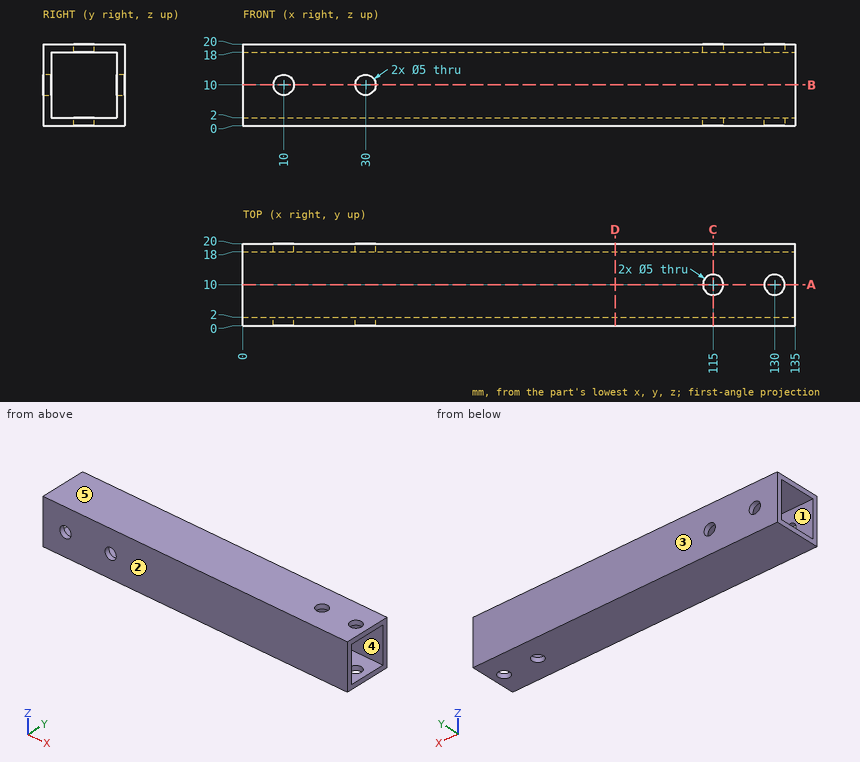
The drawing under review shows one solid part. Ordinate dimensions are in mm from its lowest x, y, z. A direction names the side the tool comes from. Round coordinates to 2 decimals unless told otherwise and drop trailing zeros. Order: outer loops, then holes, each group sorted by start corner. A loop starts at its lowest first (then second) coordinate and runs counter-clockwise, first axis right, second up. Notation, with made-up numbers: (85.5, -35) -> (111.5, -35) arc R20 ccw to (111.5, -23) -> close; hole circle Ø10 at (55.5, 44.25). An arc over 180 degrees is marked (long way). Use a Markdown table: item, result.
Q1. Tool access review of the marked faces 4 and 5: name each direction out of +Z, -Z, +X, -X, +Y, -Y from which nothing blocks a thin tool from reaching the whole face with its end or side.
Values:
| item | result |
|---|---|
| face 4 | +X, -X |
| face 5 | +Z, +X, -X, +Y, -Y |
Q2. Mouldability with a two-part tool opening along Y and no side actions: class the marked faces 1, 2 and 3 as +Y half, -Y half, draft (parallel to the pull), parting line (faces both ways), or undercut.
Values:
| item | result |
|---|---|
| face 1 | undercut |
| face 2 | -Y half |
| face 3 | +Y half |
Q3. We need section A-A on y = 10. Write out the cut boundary in (x, z), then the cut area to 3 significant figures.
Values:
| item | result |
|---|---|
| outline | (0, 0) -> (112.5, 0) -> (112.5, 2) -> (0, 2) -> close; (0, 18) -> (112.5, 18) -> (112.5, 20) -> (0, 20) -> close; (117.5, 0) -> (127.5, 0) -> (127.5, 2) -> (117.5, 2) -> close; (117.5, 18) -> (127.5, 18) -> (127.5, 20) -> (117.5, 20) -> close; (132.5, 0) -> (135, 0) -> (135, 2) -> (132.5, 2) -> close; (132.5, 18) -> (135, 18) -> (135, 20) -> (132.5, 20) -> close |
| area | 500 mm^2 |
Q4. We need section C-C on x = 115. Write out the cut boundary in (y, z), then the cut area to 3 significant figures.
Values:
| item | result |
|---|---|
| outline | (0, 0) -> (7.5, 0) -> (7.5, 2) -> (2, 2) -> (2, 18) -> (7.5, 18) -> (7.5, 20) -> (0, 20) -> close; (12.5, 0) -> (20, 0) -> (20, 20) -> (12.5, 20) -> (12.5, 18) -> (18, 18) -> (18, 2) -> (12.5, 2) -> close |
| area | 124 mm^2 |
Q5. We need section B-B on z = 10. Write out the cut boundary in (x, y), then the cut area to 3 significant figures.
Values:
| item | result |
|---|---|
| outline | (0, 0) -> (7.5, 0) -> (7.5, 2) -> (0, 2) -> close; (0, 18) -> (7.5, 18) -> (7.5, 20) -> (0, 20) -> close; (12.5, 0) -> (27.5, 0) -> (27.5, 2) -> (12.5, 2) -> close; (12.5, 18) -> (27.5, 18) -> (27.5, 20) -> (12.5, 20) -> close; (32.5, 0) -> (135, 0) -> (135, 2) -> (32.5, 2) -> close; (32.5, 18) -> (135, 18) -> (135, 20) -> (32.5, 20) -> close |
| area | 500 mm^2 |
Q6. For line 1 (X direction, y = 19.35, z = 10); line 2 (Y direction, x = 129, z = 7), list the stretches that pass through material, from the lowest coordinate up.
Values:
| item | result |
|---|---|
| line 1 | x = 0 to 7.5, 12.5 to 27.5, 32.5 to 135 |
| line 2 | y = 0 to 2, 18 to 20 |
Q7. We need section D-D on x = 91. Write out the cut boundary in (y, z), then the cut area to 3 significant figures.
Values:
| item | result |
|---|---|
| outline | (0, 0) -> (20, 0) -> (20, 20) -> (0, 20) -> close; hole (2, 2) -> (18, 2) -> (18, 18) -> (2, 18) -> close |
| area | 144 mm^2 |
